from build123d import *

# Parameters (mm, degrees)
SKETCH_R  = 25.5
PAD_DEPTH = 18


with BuildPart() as part:
    # Sketch → Pad (new body)
    with BuildSketch(Plane.XY):
        with BuildLine():
            ThreePointArc((-9.5, 0), (-2.782486, 2.782486), (0, 9.5))
            Line((0, 9.5), (0, 354.5))
            ThreePointArc((0, 354.5), (-2.782486, 361.217515), (-9.500001, 364))
            Line((-9.500001, 364), (-454.5, 364))
            ThreePointArc((-454.5, 364), (-461.217514, 361.217514), (-464, 354.5))
            Line((-464, 354.5), (-464, 9.5))
            ThreePointArc((-464, 9.5), (-461.217514, 2.782485), (-454.5, 0))
            Line((-454.5, 0), (-9.5, 0))
        make_face()
        with Locations((-418, 318)):
            Circle(SKETCH_R, mode=Mode.SUBTRACT)
        with BuildLine():
            ThreePointArc((-205, 39.5), (-214.5, 30), (-205, 20.5))
            Line((-205, 20.5), (-30.5, 20.5))
            ThreePointArc((-30.5, 20.5), (-21, 30), (-30.5, 39.5))
            Line((-205, 39.5), (-30.5, 39.5))
        make_face(mode=Mode.SUBTRACT)
        with BuildLine():
            ThreePointArc((-90.75, 77.5), (-100.25, 68), (-90.75, 58.5))
            Line((-90.75, 58.5), (-30.5, 58.5))
            ThreePointArc((-30.5, 58.5), (-21, 68), (-30.5, 77.5))
            Line((-90.75, 77.5), (-30.5, 77.5))
        make_face(mode=Mode.SUBTRACT)
        with BuildLine():
            ThreePointArc((-205, 115.5), (-214.5, 106), (-205, 96.5))
            Line((-205, 96.5), (-30.5, 96.5))
            ThreePointArc((-30.5, 96.5), (-21, 106), (-30.5, 115.5))
            Line((-205, 115.5), (-30.5, 115.5))
        make_face(mode=Mode.SUBTRACT)
        with BuildLine():
            ThreePointArc((-90.75, 153.5), (-100.25, 144), (-90.75, 134.5))
            Line((-90.75, 134.5), (-30.5, 134.5))
            ThreePointArc((-30.5, 134.5), (-21, 144), (-30.5, 153.5))
            Line((-90.75, 153.5), (-30.5, 153.5))
        make_face(mode=Mode.SUBTRACT)
        with BuildLine():
            ThreePointArc((-205, 191.5), (-214.5, 182), (-205, 172.5))
            Line((-205, 172.5), (-30.5, 172.5))
            ThreePointArc((-30.5, 172.5), (-21, 182), (-30.5, 191.5))
            Line((-205, 191.5), (-30.5, 191.5))
        make_face(mode=Mode.SUBTRACT)
        with BuildLine():
            ThreePointArc((-90.75, 229.5), (-100.25, 220), (-90.75, 210.5))
            Line((-90.75, 210.5), (-30.5, 210.5))
            ThreePointArc((-30.5, 210.5), (-21, 220), (-30.5, 229.5))
            Line((-90.75, 229.5), (-30.5, 229.5))
        make_face(mode=Mode.SUBTRACT)
        with BuildLine():
            ThreePointArc((-205, 267.5), (-214.5, 258), (-205, 248.5))
            Line((-205, 248.5), (-30.5, 248.5))
            ThreePointArc((-30.5, 248.5), (-21, 258), (-30.5, 267.5))
            Line((-205, 267.5), (-30.5, 267.5))
        make_face(mode=Mode.SUBTRACT)
        with BuildLine():
            ThreePointArc((-90.75, 305.5), (-100.25, 296), (-90.75, 286.5))
            Line((-90.75, 286.5), (-30.5, 286.5))
            ThreePointArc((-30.5, 286.5), (-21, 296), (-30.5, 305.5))
            Line((-90.75, 305.5), (-30.5, 305.5))
        make_face(mode=Mode.SUBTRACT)
        with BuildLine():
            ThreePointArc((-259, 20.5), (-249.5, 30), (-259, 39.5))
            Line((-259, 39.5), (-433.5, 39.5))
            ThreePointArc((-433.5, 39.5), (-443, 30), (-433.5, 20.5))
            Line((-259, 20.5), (-433.5, 20.5))
        make_face(mode=Mode.SUBTRACT)
        with BuildLine():
            ThreePointArc((-433.5, 77.5), (-443, 68), (-433.5, 58.5))
            Line((-433.5, 58.5), (-373.25, 58.5))
            ThreePointArc((-373.25, 58.5), (-363.75, 68), (-373.25, 77.5))
            Line((-433.5, 77.5), (-373.25, 77.5))
        make_face(mode=Mode.SUBTRACT)
        with BuildLine():
            ThreePointArc((-319.25, 77.5), (-328.75, 68), (-319.25, 58.5))
            Line((-319.25, 58.5), (-144.75, 58.5))
            ThreePointArc((-144.75, 58.5), (-135.25, 68), (-144.75, 77.5))
            Line((-319.25, 77.5), (-144.75, 77.5))
        make_face(mode=Mode.SUBTRACT)
        with BuildLine():
            ThreePointArc((-433.5, 115.5), (-443, 106), (-433.5, 96.5))
            Line((-433.5, 96.5), (-259, 96.5))
            ThreePointArc((-259, 96.5), (-249.5, 106), (-259, 115.5))
            Line((-433.5, 115.5), (-259, 115.5))
        make_face(mode=Mode.SUBTRACT)
        with BuildLine():
            ThreePointArc((-319.25, 153.5), (-328.75, 144), (-319.25, 134.5))
            Line((-319.25, 134.5), (-144.75, 134.5))
            ThreePointArc((-144.75, 134.5), (-135.25, 144), (-144.75, 153.5))
            Line((-319.25, 153.5), (-144.75, 153.5))
        make_face(mode=Mode.SUBTRACT)
        with BuildLine():
            ThreePointArc((-373.25, 134.5), (-363.75, 144), (-373.25, 153.5))
            Line((-373.25, 153.5), (-433.5, 153.5))
            ThreePointArc((-433.5, 153.5), (-443, 144), (-433.5, 134.5))
            Line((-373.25, 134.5), (-433.5, 134.5))
        make_face(mode=Mode.SUBTRACT)
        with BuildLine():
            ThreePointArc((-259, 172.5), (-249.5, 182), (-259, 191.5))
            Line((-259, 191.5), (-433.5, 191.5))
            ThreePointArc((-433.5, 191.5), (-443, 182), (-433.5, 172.5))
            Line((-259, 172.5), (-433.5, 172.5))
        make_face(mode=Mode.SUBTRACT)
        with BuildLine():
            ThreePointArc((-144.75, 210.5), (-135.25, 220), (-144.75, 229.5))
            Line((-144.75, 229.5), (-319.25, 229.5))
            ThreePointArc((-319.25, 229.5), (-328.75, 220), (-319.25, 210.5))
            Line((-144.75, 210.5), (-319.25, 210.5))
        make_face(mode=Mode.SUBTRACT)
        with BuildLine():
            ThreePointArc((-373.25, 210.5), (-363.75, 220), (-373.25, 229.5))
            Line((-373.25, 229.5), (-433.5, 229.5))
            ThreePointArc((-433.5, 229.5), (-443, 220), (-433.5, 210.5))
            Line((-373.25, 210.5), (-433.5, 210.5))
        make_face(mode=Mode.SUBTRACT)
        with BuildLine():
            ThreePointArc((-259, 248.5), (-249.5, 258), (-259, 267.5))
            Line((-259, 267.5), (-433.5, 267.5))
            ThreePointArc((-433.5, 267.5), (-443, 258), (-433.5, 248.5))
            Line((-259, 248.5), (-433.5, 248.5))
        make_face(mode=Mode.SUBTRACT)
        with BuildLine():
            ThreePointArc((-319.25, 305.5), (-328.75, 296), (-319.25, 286.5))
            Line((-319.25, 286.5), (-144.75, 286.5))
            ThreePointArc((-144.75, 286.5), (-135.25, 296), (-144.75, 305.5))
            Line((-319.25, 305.5), (-144.75, 305.5))
        make_face(mode=Mode.SUBTRACT)
        with BuildLine():
            ThreePointArc((-30.5, 324.5), (-21, 334), (-30.5, 343.5))
            Line((-30.5, 343.5), (-205, 343.5))
            ThreePointArc((-205, 343.5), (-214.5, 334), (-205, 324.5))
            Line((-30.5, 324.5), (-205, 324.5))
        make_face(mode=Mode.SUBTRACT)
        with BuildLine():
            ThreePointArc((-259, 324.5), (-249.5, 334), (-259, 343.5))
            Line((-259, 343.5), (-362, 343.5))
            ThreePointArc((-362, 343.5), (-371.5, 334), (-362, 324.5))
            Line((-259, 324.5), (-362, 324.5))
        make_face(mode=Mode.SUBTRACT)
    extrude(amount=PAD_DEPTH)


solid = part.part
Design review of the part built by this model. Coordinates are the model's own, in mm. Round coordinates to 2 decimals unless told otherwise and drop trailing zeros. Write each loop counter-clockwise with the first axis right and the second up, starting at its lowest first coordinate (ties: lowest second). Pieces come first, ordered by that corner, then holes. Notation, with made-up numbers: M 7,86 L 26,86 A17 cw 26,109 Z; hole C 10,85.5 d4. An arc over 180 degrees is marked long. One line per item, written item: value. Start each with the question number.
1. To check wall thickness, follow probe 1 along Y at (x, z) = (-350, 16); probe 2 along Y at (x, z) = (-236, 10.25); probe 3 along X at (y, z) = (214, 8.75). State the ranges of each line that lie inside material, in increasing order. Write a range as from..to.
2. Take a section at A-A on y = 182. State the section outline as (x, z) points.
3. Take a section at C-C on y = 68. State the section outline as (x, z) points, then the cut area to 3 significant figures.
4. Take a section at D-D on y = 318. State the section outline as (x, z) points, then the cut area to 3 significant figures.
5. Draft analysis for pull direction X (two halves, no side actions). For faces 1 (the face through (-214.498, 30.209, 8.874)), 2 (the face through (-461.291, 2.857, 8.874)), 3 (the face through (0, 180, 9)), state which applies: pulls with the +X half, pulls with the -X half, needs draft (parallel to the pull), parting line crosses it, or undercut.
6. Take a section at B-B on x = -384. State how many separate pieces and enclosed holes the cut face has, then the cut area to 3 significant figures.
Computed:
1. probe 1: y = 0..20.5, 39.5..96.5, 115.5..172.5, 191.5..248.5, 267.5..324.5, 343.5..364
1. probe 2: y = 0..58.5, 77.5..134.5, 153.5..210.5, 229.5..286.5, 305.5..364
1. probe 3: x = -464..-440.87, -365.88..-326.62, -137.38..-98.12, -23.13..0
2. outline: M -464,0 L -443,0 L -443,18 L -464,18 Z; M -249.5,0 L -214.5,0 L -214.5,18 L -249.5,18 Z; M -21,0 L 0,0 L 0,18 L -21,18 Z
3. outline: M -464,0 L -443,0 L -443,18 L -464,18 Z; M -363.75,0 L -328.75,0 L -328.75,18 L -363.75,18 Z; M -135.25,0 L -100.25,0 L -100.25,18 L -135.25,18 Z; M -21,0 L 0,0 L 0,18 L -21,18 Z
3. area: 2,020 mm²
4. outline: M -464,0 L -443.5,0 L -443.5,18 L -464,18 Z; M -392.5,0 L 0,0 L 0,18 L -392.5,18 Z
4. area: 7,430 mm²
5. face 1: undercut
5. face 2: pulls with the -X half
5. face 3: pulls with the +X half
6. separate pieces: 8
6. enclosed holes: 0
6. area: 4,160 mm²
